Model file for the job. Use its own axes, mm. Face numbers are marked on the shaded views. A direction names the side the tool comes from. Coordinates: 2 decimals unless noted, no trailing zeros. Write each loop counter-clockwise with the first axis right and the second up, starting at its lowest first coordinate (ties: lowest second). Pieces come first, ordered by that corner, then holes.
Q1. Band-saw the part on A-A, the plane y = -0.25. Write the cut outline in (x, z).
Q2. Band-saw the part on B-B, the plane x = 2. Write the cut outline in (y, z), plus the area to 3 significant figures.
Q3. Pin check, flat tips, straight feed: P1, Ø1.1, axis at y = 0, z = -6, coming from the +X side; P2, Ø3, axis at x = 1, z = -4.5, coming from the -Y side; P3, Ø1, axis at x = 2.5, z = -4, coming from the +Y side; P4, Ø0.5, axis at y = 0, z = -4.5, coming from the -X side. Stop position of each tip, or through.
Q4. Drill centre lines: probe 1 along Z at (x, y) = (1.5, -1.5); probe 2 along X at (y, z) = (0.35, -6.5); probe 3 along Y at (x, z) = (0.25, -6.5). Where is each one in solid material? Low to high.
Q5. Band-saw the part on C-C, the plane z = -6. Write the cut outline in (x, y), plus the area to 3 significant figures.
Q6. Which spindle directions (+Z, -Z, +X, -X, +Y, -Y) get a long thin tool onto all of the face, cutting with end or side? Do the marked faces 1, 2 and 3. Say none if no direction does.
Q7. Band-saw the part on D-D, the plane y = 0.8. Write the cut outline in (x, z), plus the area to 3 significant figures.
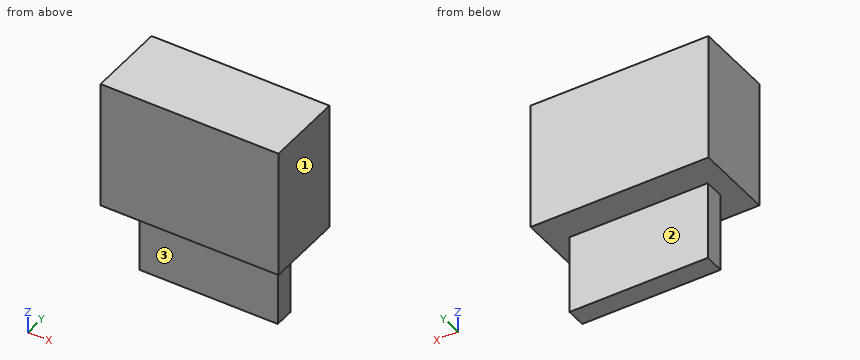
from build123d import *

# Parameters (mm, degrees)
SKETCH1_W           = 9
SKETCH1_H           = 4
BOSS_EXTRUDE1_DEPTH = 3.25
SKETCH2_W           = 7
SKETCH2_H           = 1
BOSS_EXTRUDE2_DEPTH = 4


with BuildPart() as part:
    # Sketch1 → Boss-Extrude1 (new, symmetric)
    with BuildSketch(Plane.XY):
        Rectangle(SKETCH1_W, SKETCH1_H)
    extrude(amount=BOSS_EXTRUDE1_DEPTH, both=True)

    # Sketch2 → Boss-Extrude2 (add)
    with BuildSketch(Plane(origin=(0, 0, -3.25), x_dir=(-1, 0, 0), z_dir=(0, 0, -1))):
        Rectangle(SKETCH2_W, SKETCH2_H)
    extrude(amount=BOSS_EXTRUDE2_DEPTH)


solid = part.part
Answer sheet:
1. outline: (-4.5, -3.25) - (-3.5, -3.25) - (-3.5, -7.25) - (3.5, -7.25) - (3.5, -3.25) - (4.5, -3.25) - (4.5, 3.25) - (-4.5, 3.25) - close
2. outline: (-2, -3.25) - (-0.5, -3.25) - (-0.5, -7.25) - (0.5, -7.25) - (0.5, -3.25) - (2, -3.25) - (2, 3.25) - (-2, 3.25) - close
2. area: 30.0 mm2
3. P1: stops at x = 3.5
3. P2: stops at y = -2
3. P3: stops at y = 0.5
3. P4: stops at x = -3.5
4. probe 1: z = -3.25 to 3.25
4. probe 2: x = -3.5 to 3.5
4. probe 3: y = -0.5 to 0.5
5. outline: (-3.5, -0.5) - (3.5, -0.5) - (3.5, 0.5) - (-3.5, 0.5) - close
5. area: 7.00 mm2
6. face 1: +Z, -Z, +X, +Y, -Y
6. face 2: -Z, +X, -X, +Y
6. face 3: -Z, +X, -X, -Y
7. outline: (-4.5, -3.25) - (4.5, -3.25) - (4.5, 3.25) - (-4.5, 3.25) - close
7. area: 58.5 mm2
